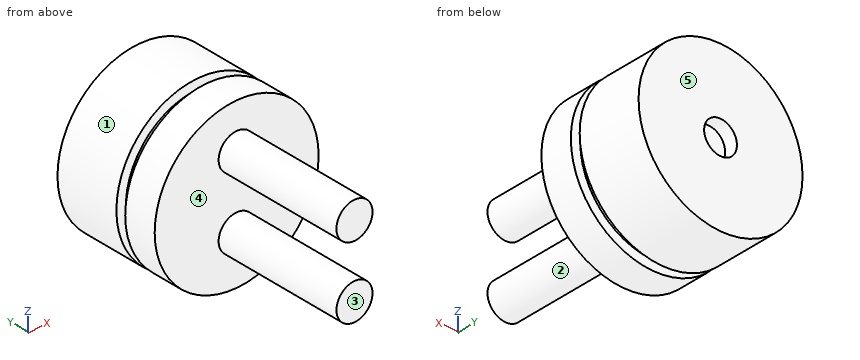
Autodesk Inventor part; units mm, degrees
ref_plane "YZ Plane" through (0, 0, 0) normal (1, 0, 0) x (0, 1, 0)
ref_plane "XZ Plane" through (0, 0, 0) normal (0, 1, 0) x (-1, 0, 0)
ref_plane "XY Plane" through (0, 0, 0) normal (0, 0, 1) x (1, 0, 0)
sketch "Sketch1" plane through (0, 0, 0) normal (0, 1, 0) x (-1, 0, 0)
  circle A0 centre (0, 0) radius 25
  dimension "d0" = 50
extrude "Extrusion1" add sketch "Sketch1" along normal blind 10
sketch "Sketch2" plane through (0, 10, 0) normal (0, 1, 0) x (1, 0, 0)
  circle A0 centre (0, 0) radius 22.1112
extrude "Extrusion2" add sketch "Sketch2" along normal blind 3
sketch "Sketch3" plane through (0, 13, 0) normal (0, 1, 0) x (1, 0, 0)
  circle A0 centre (0, 0) radius 25
extrude "Extrusion3" add sketch "Sketch3" along normal blind 20
sketch "Sketch4" plane through (0, 0, 0) normal (0, -1, 0) x (1, 0, 0)
  circle A0 centre (0, 11.3406) radius 5.5026
  circle A1 centre (0, -10.3381) radius 5.5026
  point P0 (0, 0)
extrude "Extrusion4" add sketch "Sketch4" along normal blind 40
sketch "Sketch5" plane through (0, 33, 0) normal (0, 1, 0) x (1, 0, 0)
  circle A0 centre (0, 0) radius 25
hole "Hole1" at (0, 33, 0) direction (0, -1, 0) diameter 10 depth 4
properties part number "buzzer now"
Work out the finished part from the listing and answer in its coordinate system (mm). Face numbers are marked on the shaded views. A direction names the side the tool comes from. Give positions to 0.01 mm unless a question says otherwise; leave off trailing zeros. Loops run counter-clockwise (first coordinate to the right, second up) from the corner with the lowest first, then second, coordinate; pieces in that order, holes last. Notation, with made-up numbers: M 26,4 L 67,4 A17 ccw 67,25 Z; hole C -36.75,74.25 d3. An arc over 180 degrees is marked long. One line per item, written item: value. Start each with the question number.
1. Find section D-D (y = -35). Give the vertices of the cut face in (x, z), and give its area (3 significant figures).
2. Which of the six approach directions +Z, -Z, +X, -X, +Y, -Y give full straight-line access (tool end or side, diameter ignored) to the marked faces 4 and 5?
3. Find the intervals of material crossed by probe 1 along Y at (x, z) = (23.5, 0); probe 2 along Z at (x, y) = (0, 31.35), in increasing order.
4. Determine the mould class of the marked faces 1, 2 and 3 for opening direction Z: released by +Z, released by -Z, zero draft, split by the parting line, or undercut.
5. Find section B-B (x = 0). Give the vertices of the cut face in (y, z).
6. Find section C-C (y = 1.5). Give the vertices of the cut face in (x, z).
7. Each of these flat-tipped pins is pushed along its axis until it touches: P1, Ø3, axis at y = -19.5, z = 6.5, coming from the +X side; P2, Ø5, axis at x = 9, y = -2, coming from the +Z side; P3, Ø1.5, axis at x = -8.5, y = 1, coming from the -Z side; P4, Ø8, axis at x = 1.5, z = -0.5, coming from the +Y side. Where does it stop, or does it pass through?
8. Find section A-A (z = 0). Give the vertices of the cut face in (x, y).
Reported:
1. outline: C 0,-10.34 d11.01; C 0,11.34 d11.01
1. area: 190 mm²
2. face 4: -Y
2. face 5: +Z, -Z, +X, -X, +Y
3. probe 1: y = 0 to 10, 13 to 33
3. probe 2: z = -25 to -5, 5 to 25
4. face 1: split by the parting line
4. face 2: undercut
4. face 3: zero draft
5. outline: M -40,-15.84 L 0,-15.84 L 0,-25 L 10,-25 L 10,-22.11 L 13,-22.11 L 13,-25 L 33,-25 L 33,-5 L 29,-5 L 29,5 L 33,5 L 33,25 L 13,25 L 13,22.11 L 10,22.11 L 10,25 L 0,25 L 0,16.84 L -40,16.84 L -40,5.84 L 0,5.84 L 0,-4.84 L -40,-4.84 Z
6. outline: C 0,0 d50
7. P1: stops at x = 4.37
7. P2: stops at z = 23.85
7. P3: stops at z = -23.77
7. P4: stops at y = 33
8. outline: M -25,0 L 25,0 L 25,10 L 22.11,10 L 22.11,13 L 25,13 L 25,33 L 5,33 L 5,29 L -5,29 L -5,33 L -25,33 L -25,13 L -22.11,13 L -22.11,10 L -25,10 Z
